Source: CAD feature listing. Evaluate the final solid. Frame: model axes, mm. Face numbers are marked on the shaded views. A direction names the side the tool comes from. Give positions to 0.01 mm unless a question says otherwise; leave off trailing zeros. Loops run counter-clockwise (first coordinate to the right, second up) from the corner with the lowest first, then second, coordinate; pieces in that order, holes last. Notation, with made-up numbers: M 24,-35 L 56,-35 A20 cw 56,-21 Z; hole C -23,1.25 d11. An arc over 180 degrees is marked long. Answer in a Markdown table with one row per item.
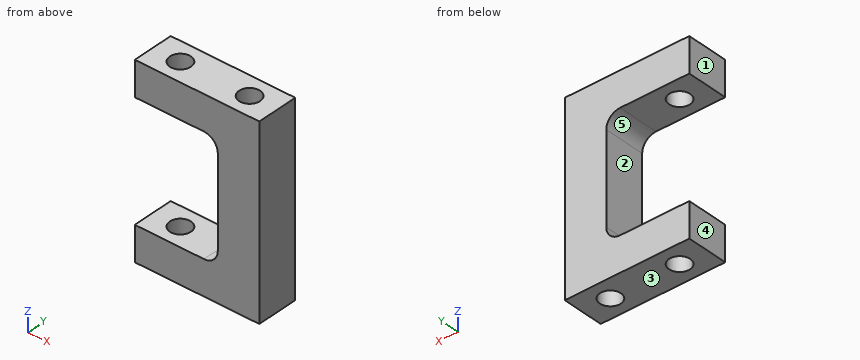
```python
from build123d import *

# Parameters (mm, degrees)
SKETCH1_W           = 90
SKETCH1_H           = 30
BOSS_EXTRUDE1_DEPTH = 25
SKETCH2_W           = 110
SKETCH2_H           = 30
BOSS_EXTRUDE2_DEPTH = 30
BOSS_EXTRUDE3_START = -90
SKETCH3_W           = 25
SKETCH3_H           = 30
BOSS_EXTRUDE3_DEPTH = 90
SKETCH4_R           = 7.6
CUT_EXTRUDE1_DEPTH  = 144.090880213
FILLET1_R           = 10


with BuildPart() as part:
    # Sketch1 → Boss-Extrude1 (new body)
    with BuildSketch(Plane.XY):
        Rectangle(SKETCH1_W, SKETCH1_H)
    extrude(amount=BOSS_EXTRUDE1_DEPTH)

    # Sketch2 → Boss-Extrude2 (add)
    with BuildSketch(Plane(origin=(45, 0, 0), x_dir=(0, 0, -1), z_dir=(1, 0, 0))):
        with Locations((-55, 0)):
            Rectangle(SKETCH2_W, SKETCH2_H)
    extrude(amount=-BOSS_EXTRUDE2_DEPTH)

    # Sketch3 → Boss-Extrude3 (add)
    with BuildSketch(Plane(origin=(45, 0, 0), x_dir=(0, 0, -1), z_dir=(1, 0, 0)).offset(BOSS_EXTRUDE3_START)):
        with Locations((-122.5, 0)):
            Rectangle(SKETCH3_W, SKETCH3_H)
    extrude(amount=BOSS_EXTRUDE3_DEPTH)

    # Sketch4 → Cut-Extrude1 (cut, through all)
    with BuildSketch(Plane(origin=(0, 0, 0), x_dir=(-1, 0, 0), z_dir=(0, 0, -1))):
        with Locations((25, 0)):
            Circle(SKETCH4_R)
        with Locations((-25, 0)):
            Circle(SKETCH4_R)
    extrude(amount=-CUT_EXTRUDE1_DEPTH, mode=Mode.SUBTRACT)

    # Fillet1
    fillet1_edges = [part.edges().sort_by_distance(p)[0] for p in [
        (15, 0, 25),
        (15, 0, 110),
    ]]
    fillet(fillet1_edges, radius=FILLET1_R)


solid = part.part
```
Q1. Section query B-B (y = 0). Output: boundary loops of the cut face in (x, z).
Values follow:
| item | result |
|---|---|
| outline | M -45,0 L -32.6,0 L -32.6,25 L -45,25 Z; M -45,110 L -32.6,110 L -32.6,135 L -45,135 Z; M -17.4,0 L 17.4,0 L 17.4,135 L -17.4,135 L -17.4,110 L 5,110 A10 cw 15,100 L 15,35 A10 cw 5,25 L -17.4,25 Z; M 32.6,0 L 45,0 L 45,135 L 32.6,135 Z |
Q2. Section query C-C (x = 25). Output: boundary loops of the cut face in (y, z).
Values follow:
| item | result |
|---|---|
| outline | M -15,0 L -7.6,0 L -7.6,135 L -15,135 Z; M 7.6,0 L 15,0 L 15,135 L 7.6,135 Z |
Q3. Mould query, pull axis Z, two halves, no side actions, for the marked faces 3, 4 and 5. Classes: +Z half, -Z half, draft (parallel to the pull), parting line (faces both ways), or undercut.
Values follow:
| item | result |
|---|---|
| face 3 | -Z half |
| face 4 | draft |
| face 5 | undercut |
Q4. Reachability of the marked faces 1 and 2 from +Z, -Z, +X, -X, +Y, -Y: full face, straight path, thin tool, end or side. Return the list, or none.
Values follow:
| item | result |
|---|---|
| face 1 | +Z, -Z, -X, +Y, -Y |
| face 2 | -X, +Y, -Y |
Q5. Ray query, probe 1 along Y at (x, z) = (-25, 5.75); probe 2 along Z at (x, y) = (-37, -5); probe 3 along X at (y, z) = (0.25, 82). Return the intervals inside material, ascending. Write a range as from..to.
Values follow:
| item | result |
|---|---|
| probe 1 | -15..-7.6, 7.6..15 |
| probe 2 | 0..25, 110..135 |
| probe 3 | 15..17.4, 32.6..45 |
Q6. Section query D-D (z = 88.5). Output: boundary loops of the cut face in (x, y).
Values follow:
| item | result |
|---|---|
| outline | M 15,-15 L 45,-15 L 45,15 L 15,15 Z; hole C 25,0 d15.2 |
Q7. Section query A-A (x = -25). Output: boundary loops of the cut face in (y, z).
Values follow:
| item | result |
|---|---|
| outline | M -15,0 L -7.6,0 L -7.6,25 L -15,25 Z; M -15,110 L -7.6,110 L -7.6,135 L -15,135 Z; M 7.6,0 L 15,0 L 15,25 L 7.6,25 Z; M 7.6,110 L 15,110 L 15,135 L 7.6,135 Z |
Q8. Contact query for flat-ended pins moving along their axis: pin 1 Ø3 at (y, z) = (10.5, 106) entering from -X; pin 2 Ø9 at (y, z) = (-6, 51.5) entering from -X. Output: stop coordinate, or through.
Values follow:
| item | result |
|---|---|
| pin 1 | x = 11.61 |
| pin 2 | x = 15 |
